```python
from build123d import *

# Parameters (mm, degrees)
EXTRUDE_DEPTH               = 5
EXTRUDE001_DEPTH            = 5
THICKNESS_T                 = 1
BOX_W                       = 12
BOX_H                       = 31
BOX_DEPTH                   = 15
BOX001_W                    = 13
BOX001_H                    = 34
BOX001_DEPTH                = 14
CYLINDER001_W               = 48
CYLINDER001_H               = 15
CYLINDER001_ANGLE           = 60
CYLINDER001_PLACEMENT_ANGLE = 60
CYLINDER_W                  = 51
CYLINDER_H                  = 15
CYLINDER_ANGLE              = 60
CYLINDER_PLACEMENT_ANGLE    = 60
CUT002_ROLL_ANGLE           = 157.1428266503
CUT002_PITCH_ANGLE          = -35.3174864898
CUT002_PLACEMENT_ANGLE      = -150.7827400319


with BuildPart() as extrude_body:
    with BuildSketch(Plane(origin=(8.5, 45, 6), x_dir=(1, 0, 0), z_dir=(0, 1, 0))):
        with BuildLine():
            Line((5, 4), (-5, 4))
            Line((-5, 4), (-5, -3.1421356237))
            ThreePointArc((-5, -3.1421356237), (-2.5365296809, -3.7839783948), (0, -4))
            ThreePointArc((0, -4), (2.5365296809, -3.7839783948), (5, -3.1421356237))
            Line((5, -3.1421356237), (5, 4))
        make_face()
    extrude(amount=EXTRUDE_DEPTH)


with BuildPart() as extrude001:
    with BuildSketch(Plane(origin=(8.5, 45, 6), x_dir=(1, 0, 0), z_dir=(0, 1, 0))):
        with BuildLine():
            Line((5, 4), (-5, 4))
            Line((-5, 4), (-5, -3.1421356237))
            ThreePointArc((-5, -3.1421356237), (-2.5365296809, -3.7839783948), (0, -4))
            ThreePointArc((0, -4), (2.5365296809, -3.7839783948), (5, -3.1421356237))
            Line((5, -3.1421356237), (5, 4))
        make_face()
    extrude(amount=EXTRUDE001_DEPTH)


with BuildPart() as bolt_bottle_side_opening:
    # Thickness base: copy of Extrude body
    add(extrude_body.part)

    # Thickness
    thickness_openings = [bolt_bottle_side_opening.faces().sort_by_distance(p)[0] for p in [
        (8.5, 50, 5.862901),
    ]]
    offset(amount=THICKNESS_T, openings=thickness_openings)

    # Fusion: union Extrude body, Extrude001
    add(extrude_body.part)
    add(extrude001.part)


with BuildPart() as bolt_bottle_side_opening_1:
    # Fusion placement: moved
    add(bolt_bottle_side_opening.part.moved(Location((0, -7, 1))))


with BuildPart() as pullbay:
    # Box → Box (new body)
    with BuildSketch(Plane(origin=(2.5, 7, 2), x_dir=(1, 0, 0), z_dir=(0, 0, 1))):
        with Locations((6, 15.5)):
            Rectangle(BOX_W, BOX_H)
    extrude(amount=BOX_DEPTH)


with BuildPart() as cut_bay_from_case:
    # Box001 → Box001 (new body)
    with BuildSketch(Plane(origin=(2, 6, 0), x_dir=(1, 0, 0), z_dir=(0, 0, 1))):
        with Locations((6.5, 17)):
            Rectangle(BOX001_W, BOX001_H)
    extrude(amount=BOX001_DEPTH)

    # Cut001: cut pullBay
    add(pullbay.part, mode=Mode.SUBTRACT)


with BuildPart() as bottle_wall001:
    # Cylinder001 → Cylinder001 (revolve)
    with BuildSketch(Plane.XZ):
        with Locations((24, 7.5)):
            Rectangle(CYLINDER001_W, CYLINDER001_H)
    revolve(axis=Axis((0, 0, 0), (0, 0, 1)), revolution_arc=CYLINDER001_ANGLE)


with BuildPart() as bottle_wall001_1:
    # Cylinder001 placement: moved
    add(bottle_wall001.part.moved(Location((8.5, -7, 0))).rotate(Axis((8.5, -7, 0), (0, 0, 1)), CYLINDER001_PLACEMENT_ANGLE))


with BuildPart() as hole_cut_out_of_case:
    # Cylinder → Cylinder (revolve)
    with BuildSketch(Plane.XZ):
        with Locations((25.5, 7.5)):
            Rectangle(CYLINDER_W, CYLINDER_H)
    revolve(axis=Axis((0, 0, 0), (0, 0, 1)), revolution_arc=CYLINDER_ANGLE)


with BuildPart() as hole_cut_out_of_case_1:
    # Cylinder placement: moved
    add(hole_cut_out_of_case.part.moved(Location((8.5, -7, 0))).rotate(Axis((8.5, -7, 0), (0, 0, 1)), CYLINDER_PLACEMENT_ANGLE))

    # Cut: cut bottle_wall001
    add(bottle_wall001_1.part, mode=Mode.SUBTRACT)


with BuildPart() as hole_cut_out_of_case_2:
    # Cut placement: moved
    add(hole_cut_out_of_case_1.part.moved(Location((0, -2, 0))))

    # Fusion001: union cut bay from case
    add(cut_bay_from_case.part)

    # Cut002: cut bolt_bottle_side_opening
    add(bolt_bottle_side_opening_1.part, mode=Mode.SUBTRACT)


with BuildPart() as hole_cut_out_of_case_3:
    # Cut002 roll: moved
    add(hole_cut_out_of_case_2.part.rotate(Axis((0, 0, 0), (1, 0, 0)), CUT002_ROLL_ANGLE))


with BuildPart() as hole_cut_out_of_case_4:
    # Cut002 pitch: moved
    add(hole_cut_out_of_case_3.part.rotate(Axis((0, 0, 0), (0, 1, 0)), CUT002_PITCH_ANGLE))


with BuildPart() as hole_cut_out_of_case_5:
    # Cut002 placement: moved
    add(hole_cut_out_of_case_4.part.rotate(Axis((0, 0, 0), (0, 0, 1)), CUT002_PLACEMENT_ANGLE))


solid = hole_cut_out_of_case_5.part
```
Model file for the job. Use its own axes, mm. A direction names the side the tool comes from. Give positions to 0.01 mm unless a question says otherwise; leave off trailing zeros. Write each loop counter-clockwise with the first axis right and the second up, starting at its lowest first coordinate (ties: lowest second). Pieces come first, ordered by that corner, then holes. Notation, with made-up numbers: (2.25, 62) -> (49.25, 62) arc R6 cw to (49.25, 67) -> close; hole circle Ø9 at (66.25, -4.75). An arc over 180 degrees is marked (long way). Use CSV: the item, a comma, the result in double quotes. Start each with the question number.
1) Drill centre lines: L1, parallel to Z at x = -16, y = 30; L2, parallel to X at y = 4, z = 7; L3, parallel to X at y = 12.5, z = 9.5. Where is each one in solid material? Low to high.
2) Cut at A-A on y = 4. List the corners of the cut face in (x, z).
3) Cut at B-B on y = 10. List the corners of the cut face in (x, z), plus the area to 3 significant figures.
4) Two-plate mould, pull along X, no slides. Class faces 4 (the flat face through (-26.43, 33.89, 6.62)), 5 (the flat face through (-24.083, 32.393, 7.209)), 6 (the flat face through (-11.5, 19.9, 3)): released by +X, released by -X, zero draft, split by the parting line, or undercut.
5) Tool access for faces 1 (the flat face through (-37.241, 18.296, 24.227)), 2 (the flat face through (-13.07, 21.64, 3.13)), 3 (the flat face through (-20.797, 14.722, 10.471)): list every direction of +Z, -Z, +X, -X, +Y, -Y with a clear straight run to the whole face (end or side of a thin tool).
6) Pin check, flat tips, straight feed: P1, Ø3, axis at y = 15.5, z = 11.5, coming from the -X side (3 decimals); P2, Ø6, axis at y = 28, z = 1.5, coming from the -X side; P3, Ø3, axis at y = 35.5, z = -1.5, coming from the +X side. Stop position of each tip, or through.
Final values:
1,L1,"z = 4.42 to 5.28, 14.42 to 17.08"
1,L2,"x = -17.62 to -16.92, -10.61 to -7.56"
1,L3,"x = -20.34 to -19.64, -12.46 to -9.4"
2,outline,"(-22.31, 1.22) -> (-21.9, 0.86) -> (-14.31, 10.21) -> (-7.65, 4.42) -> (-17.2, -3.22) -> (-15.32, -4.87) -> (-4.17, 4.05) -> (-13.45, 12.13) -> close"
3,outline,"(-23.98, 3.3) -> (-23.56, 2.94) -> (-15.97, 12.3) -> (-6.1, 3.7) -> (-13.69, -5.65) -> (-13.28, -6.01) -> (-4.42, 4.9) -> (-15.12, 14.21) -> close"
3,area,"41.6 mm2"
4,face 4,"released by -X"
4,face 5,"undercut"
4,face 6,"released by +X"
5,face 1,"+Z, -X, -Y"
5,face 2,"none"
5,face 3,"-Y"
6,P1,"stops at x = -21.875"
6,P2,"stops at x = -19.52"
6,P3,"stops at x = 1.48"
